The figure shows three views and two pictorial views of one solid part (mm, origin at its lowest corner). Answer the questions. A direction names the side the tool comes from. Coordinates: 2 decimals unless noted, no trailing zeros. Order: outer loops, then holes, each group sorted by start corner. A loop starts at its lowest first (then second) coordinate and runs counter-clockwise, first axis right, second up. Notation, with made-up numbers: M -30,22 L 15,22 A31 cw 15,46 Z; hole C 54,50.25 d9. An arc over 180 degrees is marked long. Use a Markdown table: item, result.
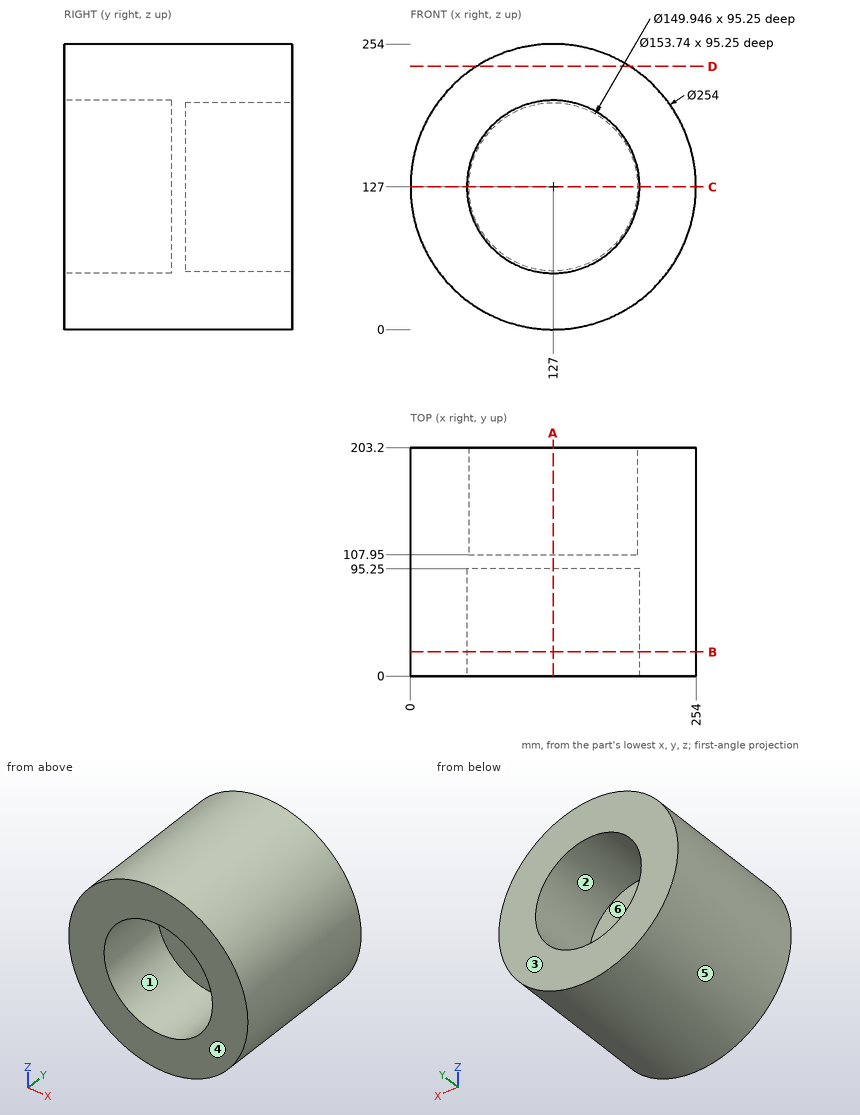
1. For a pull along Z with two mould halves and no side action, classify the marked faces 4, 5 and 6 as +Z half, -Z half, draft (parallel to the pull), parting line (faces both ways), or undercut.
Answers below:
| item | result |
|---|---|
| face 4 | draft |
| face 5 | parting line |
| face 6 | undercut |
2. Section C-C on z = 127 is taken. Determine the outline of the cut face in (x, y).
Answers below:
| item | result |
|---|---|
| outline | M 0,0 L 50.13,0 L 50.13,95.25 L 203.87,95.25 L 203.87,0 L 254,0 L 254,203.2 L 201.97,203.2 L 201.97,107.95 L 52.03,107.95 L 52.03,203.2 L 0,203.2 Z |
3. For the marked faces 1, 2 and 3, determine the directions among +Z, -Z, +X, -X, +Y, -Y from which every point of the face is accessible in a straight line to the end or side of a thin tool.
Answers below:
| item | result |
|---|---|
| face 1 | -Y |
| face 2 | +Y |
| face 3 | +Z, -Z, +X, -X, +Y |
4. Flat-ended cylindrical pins translate along their axes: P1, Ø4, axis at x = 184, z = 104, coming from the -Y side; P2, Ø3, axis at x = 171, y = 150.5, coming from the +Z side; P3, Ø1, axis at y = 65, z = 167.5, coming from the -X side. Find the tip coordinate at first contact, or state that the pin passes through.
Answers below:
| item | result |
|---|---|
| P1 | y = 95.25 |
| P2 | z = 246.68 |
| P3 | x = 6.46 |
5. Section A-A on x = 127 is taken. Determine the outline of the cut face in (y, z), then the cut area to 3 significant figures.
Answers below:
| item | result |
|---|---|
| outline | M 0,0 L 203.2,0 L 203.2,52.03 L 107.95,52.03 L 107.95,201.97 L 203.2,201.97 L 203.2,254 L 0,254 L 0,203.87 L 95.25,203.87 L 95.25,50.13 L 0,50.13 Z |
| area | 22,700 mm² |
6. Find the intervals of material crossed by probe 1 along Z at (x, y) = (127, 132.5); probe 2 along Z at (x, y) = (127, 30.5); probe 3 along Y at (x, z) = (142.5, 70), in increasing order.
Answers below:
| item | result |
|---|---|
| probe 1 | 0 to 52.03, 201.97 to 254 |
| probe 2 | 0 to 50.13, 203.87 to 254 |
| probe 3 | 95.25 to 107.95 |
7. Section D-D on z = 234 is taken. Determine the outline of the cut face in (x, y), then the cut area to 3 significant figures.
Answers below:
| item | result |
|---|---|
| outline | M 58.59,0 L 195.41,0 L 195.41,203.2 L 58.59,203.2 Z |
| area | 27,800 mm² |
8. Section B-B on y = 21.5 is taken. Determine the outline of the cut face in (x, z), then the cut area to 3 significant figures.
Answers below:
| item | result |
|---|---|
| outline | C 127,127 d254; hole C 127,127 d153.74 |
| area | 32,100 mm² |
